CAD build for the part. Positions are in the model's coordinates, mm. A direction names the side the tool comes from. Round coordinates to 2 decimals unless told otherwise and drop trailing zeros. Loops run counter-clockwise (first coordinate to the right, second up) from the corner with the lowest first, then second, coordinate; pieces in that order, holes last.
```python
from build123d import *

# Parameters (mm, degrees)
F1_DEPTH = 40.2336
F0_R     = 10.16
F2_DEPTH = 15.7734
F3_R     = 3.302


with BuildPart() as f1:
    # F0 (on Front) → F1 (new body)
    with BuildSketch(Plane.XZ):
        with BuildLine():
            ThreePointArc((-19.211791, -32.491654), (-2.338414, -22.701375), (4.320562, -4.365113))
            ThreePointArc((4.320562, -4.365113), (-2.338414, 13.971149), (-19.211791, 23.761429))
            ThreePointArc((-19.211791, 23.761429), (-52.829438, -4.365113), (-19.211791, -32.491654))
        make_face()
        with BuildLine():
            ThreePointArc((-37.702203, -9.191113), (-38.541938, -4.365113), (-37.702203, 0.460887))
            ThreePointArc((-37.702203, 0.460887), (-24.254438, 9.922387), (-10.806673, 0.460887))
            Line((-10.806673, 0.460887), (-4.885403, 0.460887))
            Line((-4.885403, 0.460887), (-4.885403, -9.191113))
            Line((-4.885403, -9.191113), (-10.806673, -9.191113))
            ThreePointArc((-10.806673, -9.191113), (-24.254438, -18.652613), (-37.702203, -9.191113))
        make_face(mode=Mode.SUBTRACT)
    extrude(amount=F1_DEPTH)

    # F0 (on Front) → F2 (join)
    with BuildSketch(Plane.XZ):
        with BuildLine():
            ThreePointArc((-19.211791, 23.761429), (-2.338414, 13.971149), (4.320562, -4.365113))
            ThreePointArc((4.320562, -4.365113), (-2.338414, -22.701375), (-19.211791, -32.491654))
            Line((-19.211791, -32.491654), (33.082327, -23.116141))
            ThreePointArc((33.082327, -23.116141), (10.670562, -4.365113), (33.082327, 14.385915))
            Line((33.082327, 14.385915), (-19.211791, 23.761429))
        make_face()
        with BuildLine():
            ThreePointArc((48.770562, -4.365113), (44.331245, 7.859062), (33.082327, 14.385915))
            ThreePointArc((33.082327, 14.385915), (10.670562, -4.365113), (33.082327, -23.116141))
            ThreePointArc((33.082327, -23.116141), (44.331245, -16.589287), (48.770562, -4.365113))
        make_face()
        with Locations((29.720562, -4.365113)):
            Circle(F0_R, mode=Mode.SUBTRACT)
    extrude(amount=F2_DEPTH)

    # F3
    f3_edges = [f1.edges().sort_by_distance(p)[0] for p in [
        (-29.297085, -40.2336, 23.761429),
    ]]
    fillet(f3_edges, radius=F3_R)


solid = f1.part
```
Item 1: Cut at C-C, the plane y = -5. State how many separate pieces and enclosed holes the cut face has, plus the area to 3 significant figures.
Answers follow:
separate pieces: 1
enclosed holes: 2
area: 3,450 mm2
Item 2: Probe line 1 (X direction, y = -6, z = 5); line 2 (X direction, y = -36.5, z = -9.5); line 3 (X direction, y = -24, z = -4.5). List the from-to ranges inside material, lowest first.
Answers follow:
line 1: x = -51.25 to -35.04, -13.46 to 25.78, 33.66 to 46.31
line 2: x = -52.36 to -37.59, -10.92 to 3.86
line 3: x = -52.83 to -38.54, -4.89 to 4.32
Item 3: Two-plate mould, pull along X, no slides. Class faces 1 (the flat face through (7.3, -7.78, 19.01)), 2 (the flat face through (-3, 0, -4)), 3 (the flat face through (-8, -20, 0.461)): released by +X, released by -X, zero draft, split by the parting line, or undercut.
Answers follow:
face 1: released by +X
face 2: zero draft
face 3: undercut
Item 4: Flat gauge pins, fed straight in: P1, Ø5, axis at x = 16.5, z = -5.5, coming from the -Y side; P2, Ø10, axis at x = 4.5, y = -10.5, coming from the +Z side; P3, Ø3, axis at y = -27, z = -2.5, coming from the -X side; P4, Ø12, axis at x = 29.72, z = -4.37, coming from the -Y side. Where does each tip first touch, or does it go through?
Answers follow:
P1: stops at y = -15.77
P2: stops at z = 20.41
P3: stops at x = -52.83
P4: passes through
Item 5: 3-axis set-ups, long thin cutter, end or side, ignore diameter. For faces 4 (the flat face through (-13, -40.234, -15)), 5 (the flat face through (-8, -20, -9.191)): which of +Z, -Z, +X, -X, +Y, -Y reach the whole face in a straight line?
Answers follow:
face 4: +Z, -Z, +X, -X, -Y
face 5: +Y, -Y
Item 6: Cut at B-B, the plane x = 25.5. Give the cut face in (y, z), plus the area to 3 significant figures.
Answers follow:
outline: (-15.77, -24.48) - (0, -24.48) - (0, -13.61) - (-15.77, -13.61) - close; (-15.77, 4.88) - (0, 4.88) - (0, 15.75) - (-15.77, 15.75) - close
area: 343 mm2
